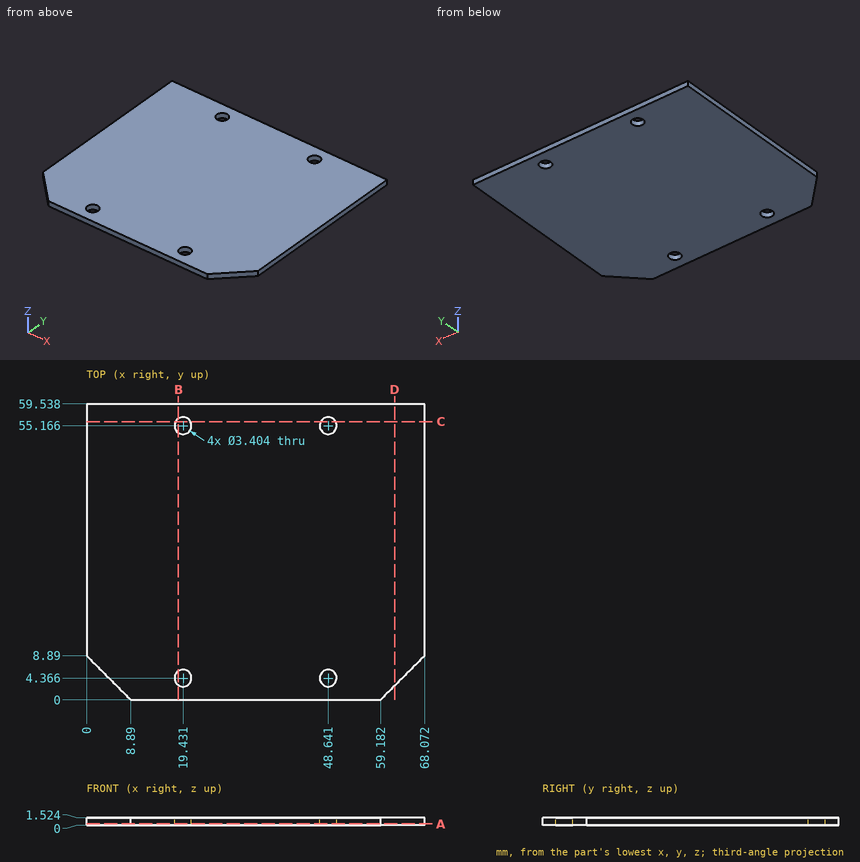
Source: three-view drawing plus pictorial views. Frame: mm from the lowest corner of the part. Give positions to 0.01 mm unless a question says otherwise; leave off trailing zeros. Order: outer loops, then holes, each group sorted by start corner. A loop starts at its lowest first (then second) coordinate and runs counter-clockwise, first axis right, second up. Notation, with made-up numbers: (4.5, 69) -> (13.5, 69) arc R26 cw to (13.5, 93) -> close; hole circle Ø1 at (26.5, -40). An arc over 180 degrees is marked (long way). Use a Markdown table: item, result.
Q1. Section A-A (z = 0.3). Return the cut outline in (x, y), and give its area (3 significant figures).
A:
| item | result |
|---|---|
| outline | (0, 8.89) -> (8.89, 0) -> (59.18, 0) -> (68.07, 8.89) -> (68.07, 59.54) -> (0, 59.54) -> close; hole circle Ø3.4 at (19.43, 4.37); hole circle Ø3.4 at (19.43, 55.17); hole circle Ø3.4 at (48.64, 4.37); hole circle Ø3.4 at (48.64, 55.17) |
| area | 3,940 mm^2 |
Q2. Material intervals for line 1 (Y direction, x = 19.5, z = 0.65); line 2 (Y direction, x = 18, z = 0.3) (1 decimal); line 3 (X direction, y = 54, z = 0.3), sorted ascending. Write a range as [from, to].
A:
| item | result |
|---|---|
| line 1 | [0, 2.67], [6.07, 53.47], [56.87, 59.54] |
| line 2 | [0, 3.4], [5.3, 54.2], [56.1, 59.5] |
| line 3 | [0, 18.19], [20.67, 47.4], [49.88, 68.07] |
Q3. Section C-C (y = 56). Return the cut outline in (x, z) (1 decimal).
A:
| item | result |
|---|---|
| outline | (0, 0) -> (17.9, 0) -> (17.9, 1.5) -> (0, 1.5) -> close; (20.9, 0) -> (47.2, 0) -> (47.2, 1.5) -> (20.9, 1.5) -> close; (50.1, 0) -> (68.1, 0) -> (68.1, 1.5) -> (50.1, 1.5) -> close |
Q4. Section D-D (x = 62). Return the cut outline in (y, z).
A:
| item | result |
|---|---|
| outline | (2.82, 0) -> (59.54, 0) -> (59.54, 1.52) -> (2.82, 1.52) -> close |
Q5. Section B-B (x = 18.5). Return the cut outline in (y, z).
A:
| item | result |
|---|---|
| outline | (0, 0) -> (2.94, 0) -> (2.94, 1.52) -> (0, 1.52) -> close; (5.79, 0) -> (53.74, 0) -> (53.74, 1.52) -> (5.79, 1.52) -> close; (56.59, 0) -> (59.54, 0) -> (59.54, 1.52) -> (56.59, 1.52) -> close |
